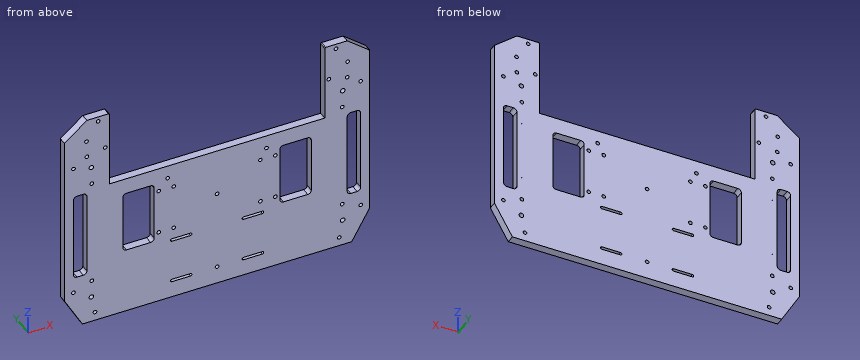
```python
from build123d import *

# Parameters (mm, degrees)
ESQUISSE3_R             = 2.55
STRUCTURE_DEPTH         = 9
ESQUISSE4_R             = 0.25
ENCOCHES_TIGES_DEPTH    = 5
ESQUISSE5_R             = 2.05
ENCODEURS_DEPTH         = 221.410979763
MOTEURS_DEPTH           = 221.410979763
MOTEURS_DEPTH_BACK      = 221.410979763
ESQUISSE6_R             = 2.05
ESQUISSE7_R             = 2.05
PATINS_DEPTH            = 221.410979763
ESQUISSE8_R             = 2.05
ACTIONNEURS_DEPTH       = 221.410979763
CONG_1_R                = 1
BATTERIE_DEPTH          = 30
ESQUISSE10_OUTSIDE_W    = 426.422
ESQUISSE10_OUTSIDE_H    = 336.422
ESQUISSE10_OUTSIDE_R    = 2.05
ESQUISSE10_OUTSIDE_R_2  = 2.55
ENL_V_MAT_EXTRU_1_DEPTH = 10
ESQUISSE11_OUTSIDE_W    = 426.422
ESQUISSE11_OUTSIDE_H    = 336.422
ESQUISSE11_OUTSIDE_R    = 2.05
ENL_V_MAT_EXTRU_2_DEPTH = 10


with BuildPart() as part:
    # Esquisse3 → structure (new body)
    with BuildSketch(Plane(origin=(0, 0, 0), x_dir=(1, 0, 0), z_dir=(0, 1, 0))):
        Polygon((150, 110), (-150, 110), (-170, 75), (-170, 0), (-170, -120), (-145, -140), (-120, -140), (-120, -53), (120, -53), (120, -140), (145, -140), (170, -120), (170, 0), (170, 75), align=None)
        with Locations(Location((-140, 80, 0), (0, 0, 270))):
            Circle(ESQUISSE3_R, mode=Mode.SUBTRACT)
        with Locations(Location((-140, -80, 0), (0, 0, 90))):
            Circle(ESQUISSE3_R, mode=Mode.SUBTRACT)
        with Locations(Location((140, -80, 0), (0, 0, 270))):
            Circle(ESQUISSE3_R, mode=Mode.SUBTRACT)
        with Locations(Location((140, 80, 0), (0, 0, 90))):
            Circle(ESQUISSE3_R, mode=Mode.SUBTRACT)
        with BuildLine():
            Line((-160, -46), (-160, 46))
            ThreePointArc((-160, 46), (-158.828427125, 48.828427125), (-156, 50))
            Line((-156, 50), (-149, 50))
            ThreePointArc((-149, 50), (-146.171572875, 48.828427125), (-145, 46))
            Line((-145, 46), (-145, -46))
            ThreePointArc((-145, -46), (-146.171572875, -48.828427125), (-149, -50))
            Line((-149, -50), (-156, -50))
            ThreePointArc((-156, -50), (-158.828427125, -48.828427125), (-160, -46))
        make_face(mode=Mode.SUBTRACT)
        with BuildLine():
            Line((-105, 0), (-105, 31))
            ThreePointArc((-105, 31), (-103.828427125, 33.828427125), (-101, 35))
            Line((-101, 35), (-74, 35))
            ThreePointArc((-74, 35), (-71.171572875, 33.828427125), (-70, 31))
            Line((-70, 31), (-70, -31))
            ThreePointArc((-70, -31), (-71.171572875, -33.828427125), (-74, -35))
            Line((-74, -35), (-101, -35))
            ThreePointArc((-101, -35), (-103.828427125, -33.828427125), (-105, -31))
            Line((-105, -31), (-105, 0))
        make_face(mode=Mode.SUBTRACT)
        with BuildLine():
            Line((156, 50), (149, 50))
            ThreePointArc((149, 50), (146.171572875, 48.828427125), (145, 46))
            Line((145, 46), (145, -46))
            ThreePointArc((145, -46), (146.171572875, -48.828427125), (149, -50))
            Line((149, -50), (156, -50))
            ThreePointArc((156, -50), (158.828427125, -48.828427125), (160, -46))
            Line((160, -46), (160, 46))
            ThreePointArc((160, 46), (158.828427125, 48.828427125), (156, 50))
        make_face(mode=Mode.SUBTRACT)
        with BuildLine():
            Line((105, 0), (105, 31))
            ThreePointArc((105, 31), (103.828427125, 33.828427125), (101, 35))
            Line((101, 35), (74, 35))
            ThreePointArc((74, 35), (71.171572875, 33.828427125), (70, 31))
            Line((70, 31), (70, -31))
            ThreePointArc((70, -31), (71.171572875, -33.828427125), (74, -35))
            Line((74, -35), (101, -35))
            ThreePointArc((101, -35), (103.828427125, -33.828427125), (105, -31))
            Line((105, -31), (105, 0))
        make_face(mode=Mode.SUBTRACT)
    extrude(amount=-STRUCTURE_DEPTH)

    # Esquisse4 → encoches_tiges (cut)
    with BuildSketch(Plane(origin=(0, 0, 0), x_dir=(1, 0, 0), z_dir=(0, 1, 0))):
        with Locations(Location((-139.5, 33.5, 0), (0, 0, 270))):
            Circle(ESQUISSE4_R)
        with Locations(Location((-139.5, -33.5, 0), (0, 0, 90))):
            Circle(ESQUISSE4_R)
        with Locations(Location((139.5, -33.5, 0), (0, 0, 270))):
            Circle(ESQUISSE4_R)
        with Locations(Location((139.5, 33.5, 0), (0, 0, 90))):
            Circle(ESQUISSE4_R)
    extrude(amount=-ENCOCHES_TIGES_DEPTH, mode=Mode.SUBTRACT)

    # Esquisse5 → encodeurs (cut, through all)
    with BuildSketch(Plane(origin=(0, 0, 0), x_dir=(1, 0, 0), z_dir=(0, 1, 0))):
        with Locations(Location((-139.5, 60, 0), (0, 0, 270))):
            Circle(ESQUISSE5_R)
        with Locations(Location((-139.5, -60, 0), (0, 0, 90))):
            Circle(ESQUISSE5_R)
        with Locations(Location((139.5, -60, 0), (0, 0, 270))):
            Circle(ESQUISSE5_R)
        with Locations(Location((139.5, 60, 0), (0, 0, 90))):
            Circle(ESQUISSE5_R)
    extrude(amount=-ENCODEURS_DEPTH, mode=Mode.SUBTRACT)

    # Esquisse6 → moteurs (cut, two sides: drawn at the far end of the back side and taken through both)
    with BuildSketch(Plane(origin=(0, 0, 0), x_dir=(1, 0, 0), z_dir=(0, 1, 0)).offset(-MOTEURS_DEPTH_BACK)):
        with Locations(Location((-65, 25.5, 0), (0, 0, 270))):
            Circle(ESQUISSE6_R)
        with Locations(Location((-48.3, 25.5, 0), (0, 0, 270))):
            Circle(ESQUISSE6_R)
        with Locations(Location((-65, -25.5, 0), (0, 0, 270))):
            Circle(ESQUISSE6_R)
        with Locations(Location((48.3, -25.5, 0), (0, 0, 270))):
            Circle(ESQUISSE6_R)
        with Locations(Location((65, -25.5, 0), (0, 0, 270))):
            Circle(ESQUISSE6_R)
        with Locations(Location((-48.3, -25.5, 0), (0, 0, 90))):
            Circle(ESQUISSE6_R)
        with Locations(Location((48.3, 25.5, 0), (0, 0, 90))):
            Circle(ESQUISSE6_R)
        with Locations(Location((65, 25.5, 0), (0, 0, 90))):
            Circle(ESQUISSE6_R)
    extrude(amount=MOTEURS_DEPTH + MOTEURS_DEPTH_BACK, mode=Mode.SUBTRACT)

    # Esquisse7 → patins (cut, through all)
    with BuildSketch(Plane(origin=(0, 0, 0), x_dir=(1, 0, 0), z_dir=(0, 1, 0))):
        with Locations(Location((0, 90, 0), (0, 0, 270))):
            Circle(ESQUISSE7_R)
        with Locations(Location((0, 0, 0), (0, 0, 270))):
            Circle(ESQUISSE7_R)
        with Locations(Location((-145, -95, 0), (0, 0, 270))):
            Circle(ESQUISSE7_R)
        with Locations(Location((145, -95, 0), (0, 0, 90))):
            Circle(ESQUISSE7_R)
    extrude(amount=-PATINS_DEPTH, mode=Mode.SUBTRACT)

    # Esquisse8 → actionneurs (cut, through all)
    with BuildSketch(Plane(origin=(0, 0, 0), x_dir=(1, 0, 0), z_dir=(0, 1, 0))):
        with Locations(Location((-132.5, -134.5, 0), (0, 0, 270))):
            Circle(ESQUISSE8_R)
        with Locations(Location((-124.5, -99.5, 0), (0, 0, 270))):
            Circle(ESQUISSE8_R)
        with Locations(Location((132.5, -134.5, 0), (0, 0, 90))):
            Circle(ESQUISSE8_R)
        with Locations(Location((124.5, -99.5, 0), (0, 0, 90))):
            Circle(ESQUISSE8_R)
        with Locations(Location((-145.5, -114, 0), (0, 0, 270))):
            Circle(ESQUISSE8_R)
        with Locations(Location((145.5, -114, 0), (0, 0, 90))):
            Circle(ESQUISSE8_R)
    extrude(amount=-ACTIONNEURS_DEPTH, mode=Mode.SUBTRACT)

    # Congé1
    cong_1_edges = [part.edges().sort_by_distance(p)[0] for p in [
        (-120, -4.5, 140),
        (120, -4.5, 140),
    ]]
    fillet(cong_1_edges, radius=CONG_1_R)

    # Esquisse9 → batterie (cut)
    with BuildSketch(Plane(origin=(0, 0, 0), x_dir=(1, 0, 0), z_dir=(0, 1, 0))):
        with BuildLine():
            ThreePointArc((29.5, 88.5), (28, 90), (29.5, 91.5))
            Line((29.5, 91.5), (50.5, 91.5))
            ThreePointArc((50.5, 91.5), (52, 90), (50.5, 88.5))
            Line((50.5, 88.5), (29.5, 88.5))
        make_face()
        with BuildLine():
            Line((-50.5, 88.5), (-29.5, 88.5))
            ThreePointArc((-29.5, 88.5), (-28, 90), (-29.5, 91.5))
            Line((-29.5, 91.5), (-50.5, 91.5))
            ThreePointArc((-50.5, 91.5), (-52, 90), (-50.5, 88.5))
        make_face()
        with BuildLine():
            Line((-50.5, 38.5), (-29.5, 38.5))
            ThreePointArc((-29.5, 38.5), (-28, 40), (-29.5, 41.5))
            Line((-29.5, 41.5), (-50.5, 41.5))
            ThreePointArc((-50.5, 41.5), (-52, 40), (-50.5, 38.5))
        make_face()
        with BuildLine():
            Line((50.5, 38.5), (29.5, 38.5))
            ThreePointArc((29.5, 38.5), (28, 40), (29.5, 41.5))
            Line((29.5, 41.5), (50.5, 41.5))
            ThreePointArc((50.5, 41.5), (52, 40), (50.5, 38.5))
        make_face()
    extrude(amount=-BATTERIE_DEPTH, mode=Mode.SUBTRACT)

    # Esquisse10 outside → Enlèv. mat.-Extru.1 (cut)
    # profile 1 of 9: a face of its own
    with BuildSketch(Plane(origin=(0, 0, 0), x_dir=(1, 0, 0), z_dir=(0, 1, 0))):
        with Locations((0, -15)):
            Rectangle(ESQUISSE10_OUTSIDE_W, ESQUISSE10_OUTSIDE_H)
        with BuildLine():
            Line((120, -53), (120, -139))
            ThreePointArc((120, -139), (120.292893219, -139.707106781), (121, -140))
            Line((121, -140), (145, -140))
            Line((145, -140), (170, -120))
            Line((170, -120), (170, 75))
            Line((170, 75), (150, 110))
            Line((150, 110), (-150, 110))
            Line((-150, 110), (-170, 75))
            Line((-170, 75), (-170, -120))
            Line((-170, -120), (-145, -140))
            Line((-145, -140), (-121, -140))
            ThreePointArc((-121, -140), (-120.292893219, -139.707106781), (-120, -139))
            Line((-120, -139), (-120, -53))
            Line((-120, -53), (120, -53))
        make_face(mode=Mode.SUBTRACT)
    # profile 2 of 9: a face of its own
    with BuildSketch(Plane(origin=(0, 0, 0), x_dir=(1, 0, 0), z_dir=(0, 1, 0))):
        with Locations(Location((-136, 100, 0), (0, 0, 270))):
            Circle(ESQUISSE10_OUTSIDE_R)
    # profile 3 of 9: a face of its own
    with BuildSketch(Plane(origin=(0, 0, 0), x_dir=(1, 0, 0), z_dir=(0, 1, 0))):
        with Locations(Location((-160, 68, 0), (0, 0, 270))):
            Circle(ESQUISSE10_OUTSIDE_R)
    # profile 4 of 9: a face of its own
    with BuildSketch(Plane(origin=(0, 0, 0), x_dir=(1, 0, 0), z_dir=(0, 1, 0))):
        with Locations(Location((-160, -85, 0), (0, 0, 270))):
            Circle(ESQUISSE10_OUTSIDE_R)
    # profile 5 of 9: a face of its own
    with BuildSketch(Plane(origin=(0, 0, 0), x_dir=(1, 0, 0), z_dir=(0, 1, 0))):
        with Locations(Location((160, -85, 0), (0, 0, 90))):
            Circle(ESQUISSE10_OUTSIDE_R)
    # profile 6 of 9: a face of its own
    with BuildSketch(Plane(origin=(0, 0, 0), x_dir=(1, 0, 0), z_dir=(0, 1, 0))):
        with Locations(Location((160, 68, 0), (0, 0, 90))):
            Circle(ESQUISSE10_OUTSIDE_R)
    # profile 7 of 9: a face of its own
    with BuildSketch(Plane(origin=(0, 0, 0), x_dir=(1, 0, 0), z_dir=(0, 1, 0))):
        with Locations(Location((136, 100, 0), (0, 0, 90))):
            Circle(ESQUISSE10_OUTSIDE_R)
    # profile 8 of 9: a face of its own
    with BuildSketch(Plane(origin=(0, 0, 0), x_dir=(1, 0, 0), z_dir=(0, 1, 0))):
        with Locations(Location((-140, 80, 0), (0, 0, 270))):
            Circle(ESQUISSE10_OUTSIDE_R_2)
    # profile 9 of 9: a face of its own
    with BuildSketch(Plane(origin=(0, 0, 0), x_dir=(1, 0, 0), z_dir=(0, 1, 0))):
        with Locations(Location((-140, -80, 0), (0, 0, 90))):
            Circle(ESQUISSE10_OUTSIDE_R_2)
    extrude(amount=-ENL_V_MAT_EXTRU_1_DEPTH, mode=Mode.SUBTRACT)

    # Esquisse11 outside → Enlèv. mat.-Extru.2 (cut)
    # profile 1 of 3: a face of its own
    with BuildSketch(Plane(origin=(0, 0, 0), x_dir=(1, 0, 0), z_dir=(0, 1, 0))):
        with Locations((0, -15)):
            Rectangle(ESQUISSE11_OUTSIDE_W, ESQUISSE11_OUTSIDE_H)
        with BuildLine():
            Line((120, -53), (120, -139))
            ThreePointArc((120, -139), (120.292893219, -139.707106781), (121, -140))
            Line((121, -140), (145, -140))
            Line((145, -140), (170, -120))
            Line((170, -120), (170, 75))
            Line((170, 75), (150, 110))
            Line((150, 110), (-150, 110))
            Line((-150, 110), (-170, 75))
            Line((-170, 75), (-170, -120))
            Line((-170, -120), (-145, -140))
            Line((-145, -140), (-121, -140))
            ThreePointArc((-121, -140), (-120.292893219, -139.707106781), (-120, -139))
            Line((-120, -139), (-120, -53))
            Line((-120, -53), (120, -53))
        make_face(mode=Mode.SUBTRACT)
    # profile 2 of 3: a face of its own
    with BuildSketch(Plane(origin=(0, 0, 0), x_dir=(1, 0, 0), z_dir=(0, 1, 0))):
        with Locations(Location((-55, -38, 0), (0, 0, 270))):
            Circle(ESQUISSE11_OUTSIDE_R)
    # profile 3 of 3: a face of its own
    with BuildSketch(Plane(origin=(0, 0, 0), x_dir=(1, 0, 0), z_dir=(0, 1, 0))):
        with Locations(Location((55, -38, 0), (0, 0, 90))):
            Circle(ESQUISSE11_OUTSIDE_R)
    extrude(amount=-ENL_V_MAT_EXTRU_2_DEPTH, mode=Mode.SUBTRACT)


solid = part.part
```
The model under review builds one solid part; all positions refer to its coordinate system, in mm. Round coordinates to 2 decimals unless told otherwise and drop trailing zeros. Order: outer loops, then holes, each group sorted by start corner. A loop starts at its lowest first (then second) coordinate and runs counter-clockwise, first axis right, second up. Notation, with made-up numbers: (9, 38.25) - (65, 38.25) arc R30 cw to (65, 76.25) - close; hole circle Ø1 at (8, 57.25). An arc over 180 degrees is marked (long way). Answer in a Markdown table with one row per item.
(1) Take a section at A-A on z = -15.5. Write out the cut boundary in (x, y).
Result set:
| item | result |
|---|---|
| outline | (-170, -9) - (-160, -9) - (-160, 0) - (-170, 0) - close; (-145, -9) - (-105, -9) - (-105, 0) - (-145, 0) - close; (-70, -9) - (70, -9) - (70, 0) - (-70, 0) - close; (105, -9) - (145, -9) - (145, 0) - (105, 0) - close; (160, -9) - (170, -9) - (170, 0) - (160, 0) - close |
(2) Take a section at D-D on x = 113.5. Write out the cut boundary in (y, z).
Result set:
| item | result |
|---|---|
| outline | (-9, -110) - (0, -110) - (0, 53) - (-9, 53) - close |
(3) Take a section at C-C on y = -1.5. Count the separate pieces of the cut face and the enclosed holes in it, plus the area to 3 significant figures.
Result set:
| item | result |
|---|---|
| separate pieces | 1 |
| enclosed holes | 46 |
| area | 54,300 mm2 |
(4) Clearance check with flat-ended pins moving along their axes: P1, Ø4.5, axis at x = -55, z = 38, coming from the +Y side; P2, Ø3.5, axis at x = 0, z = -90, coming from the -Y side; P3, Ø2, axis at x = 151.5, y = -3, coming from the +Z side; P4, Ø4.5, axis at x = 39.5, y = -3, coming from the +Z side. State where each tip first meets the part, or that it passes through.
Result set:
| item | result |
|---|---|
| P1 | stops at y = 0 |
| P2 | passes through |
| P3 | stops at z = 135.6 |
| P4 | stops at z = 53 |
(5) Take a section at B-B on x = -81. Write out the cut boundary in (y, z).
Result set:
| item | result |
|---|---|
| outline | (-9, -110) - (0, -110) - (0, -35) - (-9, -35) - close; (-9, 35) - (0, 35) - (0, 53) - (-9, 53) - close |
(6) For line 1 (Z direction, x = 65, y = -5.25); line 2 (Z direction, x = -139.5, y = -5.5); line 3 (X direction, y = -4, z = 99.5), list the stretches that pass through material, from the lowest coordinate up. Write a range as from..to.
Result set:
| item | result |
|---|---|
| line 1 | z = -110..-27.55, -23.45..23.45, 27.55..53 |
| line 2 | z = -110..-82.5, -77.5..-62.05, -57.95..57.95, 62.05..77.5, 82.5..140 |
| line 3 | x = -170..-126.55, -122.45..-120, 120..122.45, 126.55..170 |
